Verification items for the finished model (mm, model axes). A direction names the side the tool comes from. Round coordinates to 2 decimals unless told otherwise and drop trailing zeros. Write each loop counter-clockwise with the first axis right and the second up, starting at its lowest first coordinate (ties: lowest second). Pieces come first, ordered by that corner, then holes. Notation, with made-up numbers: M -3,34.5 L 41,34.5 A14 ccw 41,56.5 Z; hole C -19.5,-17 d2. An arc over 180 degrees is marked long. One line per question, with ' | ' between items. Start each with the question number.
Q1. Cross-section at B-B (x = 67). Record the boundary of the cut face in (y, z), then the cut area to 3 significant figures.
Q2. Cross-section at A-A (z = 2.25). Record the boundary of the cut face in (x, y).
Q3. Thickness scan on line 1 along Y through (x, z) = (96, -1). Record the ranges inside material, lowest first. Write a range as from..to.
Q4. Release check for a two-part mould opening along Y. For faces 1 (the face through (74, 0, -5)), 2 (the face through (74, -5, 0)), 3 (the face through (74, 0, -3.5)) record: released by +Y, released by -Y, zero draft, split by the parting line, or undercut.
Q5. Tool access check on faces 4 (the face through (74, -3.5, 0)), 5 (the face through (0, -0.1, -4.5)). Record the directions out of +Z, -Z, +X, -X, +Y, -Y that give a thin tool (end or side, any length) a straight path to the whole face; none if there is none.
from build123d import *

# Parameters (mm, degrees)
CROQUIS1_W              = 150
CROQUIS1_H              = 10
SALIENTE_EXTRUIR1_DEPTH = 10
CROQUIS2_W              = 7
CROQUIS2_H              = 7
CORTAR_EXTRUIR1_DEPTH   = 151.166574177
CROQUIS3_W              = 0.02
CROQUIS3_H              = 4.666666667
CORTAR_EXTRUIR2_DEPTH   = 0.02
CROQUIS4_W              = 0.02
CROQUIS4_H              = 4.666666667
CORTAR_EXTRUIR3_DEPTH   = 0.02
CROQUIS5_W              = 0.02
CROQUIS5_H              = 4.666666667
CORTAR_EXTRUIR4_DEPTH   = 0.02
CROQUIS6_W              = 0.02
CROQUIS6_H              = 4.666666667
CORTAR_EXTRUIR5_DEPTH   = 0.02
CROQUIS7_W              = 0.02
CROQUIS7_H              = 4.666666667
CORTAR_EXTRUIR6_DEPTH   = 0.02
CROQUIS8_W              = 0.02
CROQUIS8_H              = 4.666666667
CORTAR_EXTRUIR7_DEPTH   = 0.02
CROQUIS9_W              = 0.02
CROQUIS9_H              = 4.666666667
CORTAR_EXTRUIR8_DEPTH   = 0.02
CROQUIS10_W             = 0.02
CROQUIS10_H             = 4.666666667
CORTAR_EXTRUIR9_DEPTH   = 0.02


with BuildPart() as part:
    # Croquis1 → Saliente-Extruir1 (new body)
    with BuildSketch(Plane.XZ.offset(5)):
        with Locations((75, 0)):
            Rectangle(CROQUIS1_W, CROQUIS1_H)
    extrude(amount=-SALIENTE_EXTRUIR1_DEPTH)

    # Croquis2 → Cortar-Extruir1 (cut, through all)
    with BuildSketch(Plane.ZY):
        Rectangle(CROQUIS2_W, CROQUIS2_H)
    extrude(amount=-CORTAR_EXTRUIR1_DEPTH, mode=Mode.SUBTRACT)

    # Croquis3 → Cortar-Extruir2 (cut)
    with BuildSketch(Plane.XY.offset(5)):
        with Locations((25, 1.166666666)):
            Rectangle(CROQUIS3_W, CROQUIS3_H)
    extrude(amount=-CORTAR_EXTRUIR2_DEPTH, mode=Mode.SUBTRACT)

    # Croquis4 → Cortar-Extruir3 (cut)
    with BuildSketch(Plane.XY.offset(5)):
        with Locations((35, 1.166666666)):
            Rectangle(CROQUIS4_W, CROQUIS4_H)
    extrude(amount=-CORTAR_EXTRUIR3_DEPTH, mode=Mode.SUBTRACT)

    # Croquis5 → Cortar-Extruir4 (cut)
    with BuildSketch(Plane.XY.offset(5)):
        with Locations((45, 1.166666666)):
            Rectangle(CROQUIS5_W, CROQUIS5_H)
    extrude(amount=-CORTAR_EXTRUIR4_DEPTH, mode=Mode.SUBTRACT)

    # Croquis6 → Cortar-Extruir5 (cut)
    with BuildSketch(Plane.XY.offset(5)):
        with Locations((55, 1.166666666)):
            Rectangle(CROQUIS6_W, CROQUIS6_H)
    extrude(amount=-CORTAR_EXTRUIR5_DEPTH, mode=Mode.SUBTRACT)

    # Croquis7 → Cortar-Extruir6 (cut)
    with BuildSketch(Plane.XY.offset(5)):
        with Locations((65, 1.166666666)):
            Rectangle(CROQUIS7_W, CROQUIS7_H)
    extrude(amount=-CORTAR_EXTRUIR6_DEPTH, mode=Mode.SUBTRACT)

    # Croquis8 → Cortar-Extruir7 (cut)
    with BuildSketch(Plane.XY.offset(5)):
        with Locations((75, 1.166666666)):
            Rectangle(CROQUIS8_W, CROQUIS8_H)
    extrude(amount=-CORTAR_EXTRUIR7_DEPTH, mode=Mode.SUBTRACT)

    # Croquis9 → Cortar-Extruir8 (cut)
    with BuildSketch(Plane.XY.offset(5)):
        with Locations((85, 1.166666666)):
            Rectangle(CROQUIS9_W, CROQUIS9_H)
    extrude(amount=-CORTAR_EXTRUIR8_DEPTH, mode=Mode.SUBTRACT)

    # Croquis10 → Cortar-Extruir9 (cut)
    with BuildSketch(Plane.XY.offset(5)):
        with Locations((15, 1.166666666)):
            Rectangle(CROQUIS10_W, CROQUIS10_H)
    extrude(amount=-CORTAR_EXTRUIR9_DEPTH, mode=Mode.SUBTRACT)


solid = part.part
Determined:
1) outline: M -5,-5 L 5,-5 L 5,5 L -5,5 Z; hole M -3.5,-3.5 L 3.5,-3.5 L 3.5,3.5 L -3.5,3.5 Z | area: 51.0 mm²
2) outline: M 0,-5 L 150,-5 L 150,-3.5 L 0,-3.5 Z; M 0,3.5 L 150,3.5 L 150,5 L 0,5 Z
3) line 1: y = -5..-3.5, 3.5..5
4) face 1: zero draft | face 2: released by -Y | face 3: undercut
5) face 4: +X, -X | face 5: +Z, -Z, -X, +Y, -Y
